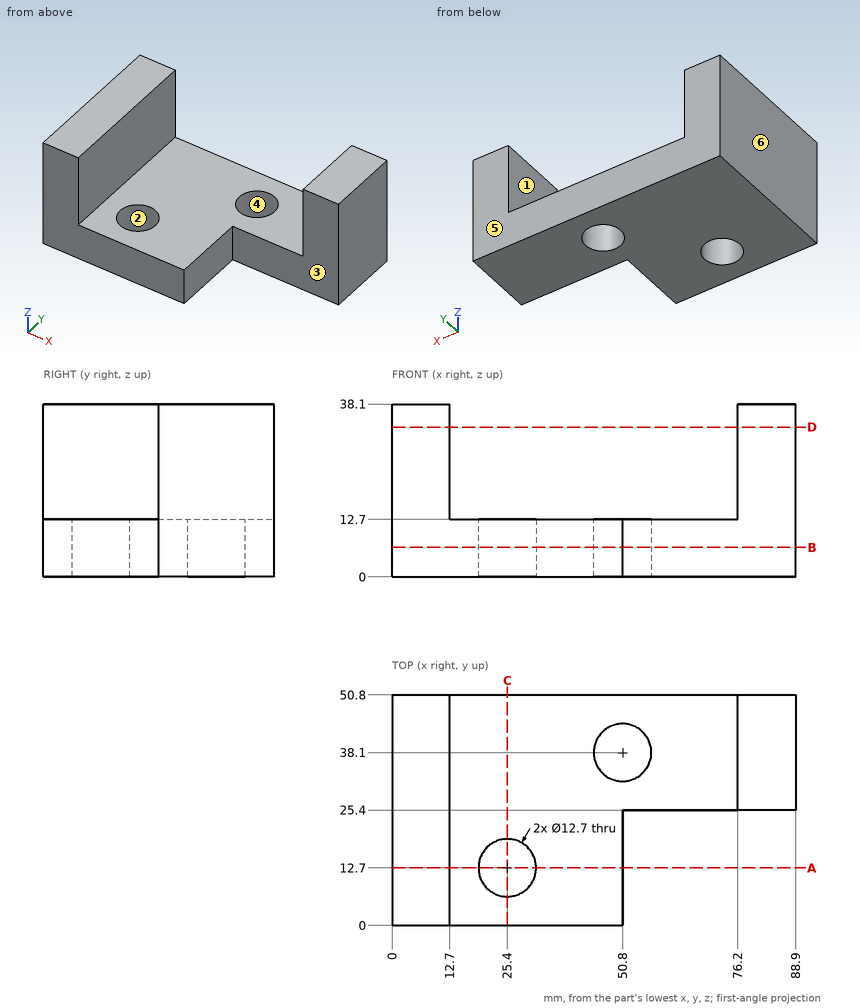
Design review of the part shown in the three views and the two pictorial views. Dimensions are in mm from the part's minimum x, y and z. A direction names the side the tool comes from. Give positions to 0.01 mm unless a question says otherwise; leave off trailing zeros. Write each loop counter-clockwise with the first axis right and the second up, starting at its lowest first coordinate (ties: lowest second). Pieces come first, ordered by that corner, then holes. Notation, with made-up numbers: (28, 28) -> (61, 28) arc R24 ccw to (61, 66) -> close; hole circle Ø7 at (40, 2.25). An arc over 180 degrees is marked (long way). Answer in a Markdown table with one row per item.
1) Clearance check with flat-ended pins moving along their axes: P1, Ø1, axis at x = 33, y = 39, coming from the +Z side; P2, Ø3, axis at x = 72, z = 4.5, coming from the -Y side; P3, Ø20.5, axis at x = 25.4, y = 12.7, coming from the -Z side; P4, Ø6, axis at y = 18.5, z = 25, coming from the +X side. State where each tip first meets the part, or that it passes through.
Worked answers:
| item | result |
|---|---|
| P1 | z = 12.7 |
| P2 | y = 25.4 |
| P3 | z = 0 |
| P4 | x = 12.7 |
2) Mouldability with a two-part tool opening along Y and no side actions: class the marked faces 4, 5 and 6 as +Y half, -Y half, draft (parallel to the pull), parting line (faces both ways), or undercut.
Worked answers:
| item | result |
|---|---|
| face 4 | undercut |
| face 5 | +Y half |
| face 6 | draft |
3) Add section B-B on z = 6.5. State the section outline as (x, y) points.
Worked answers:
| item | result |
|---|---|
| outline | (0, 0) -> (50.8, 0) -> (50.8, 25.4) -> (88.9, 25.4) -> (88.9, 50.8) -> (0, 50.8) -> close; hole circle Ø12.7 at (25.4, 12.7); hole circle Ø12.7 at (50.8, 38.1) |
4) Tool access review of the marked faces 1, 2 and 3: name each direction out of +Z, -Z, +X, -X, +Y, -Y from which nothing blocks a thin tool from reaching the whole face with its end or side.
Worked answers:
| item | result |
|---|---|
| face 1 | +Z, +Y, -Y |
| face 2 | +Z, -Z |
| face 3 | +Z, -Z, +X, -Y |
5) For L1, parallel to X at y = 27.5, z = 29.5; L2, parallel to X at y = 15.5, z = 26.5, list the stretches that pass through material, from the lowest coordinate up. Write a range as [from, to].
Worked answers:
| item | result |
|---|---|
| L1 | [0, 12.7], [76.2, 88.9] |
| L2 | [0, 12.7] |
6) Add section C-C on x = 25.4. State the section outline as (y, z) points.
Worked answers:
| item | result |
|---|---|
| outline | (0, 0) -> (6.35, 0) -> (6.35, 12.7) -> (0, 12.7) -> close; (19.05, 0) -> (50.8, 0) -> (50.8, 12.7) -> (19.05, 12.7) -> close |
7) Add section D-D on z = 33. State the section outline as (x, y) points.
Worked answers:
| item | result |
|---|---|
| outline | (0, 0) -> (12.7, 0) -> (12.7, 50.8) -> (0, 50.8) -> close; (76.2, 25.4) -> (88.9, 25.4) -> (88.9, 50.8) -> (76.2, 50.8) -> close |
8) Add section A-A on y = 12.7. State the section outline as (x, z) points, plus the area to 3 significant figures.
Worked answers:
| item | result |
|---|---|
| outline | (0, 0) -> (19.05, 0) -> (19.05, 12.7) -> (12.7, 12.7) -> (12.7, 38.1) -> (0, 38.1) -> close; (31.75, 0) -> (50.8, 0) -> (50.8, 12.7) -> (31.75, 12.7) -> close |
| area | 806 mm² |
